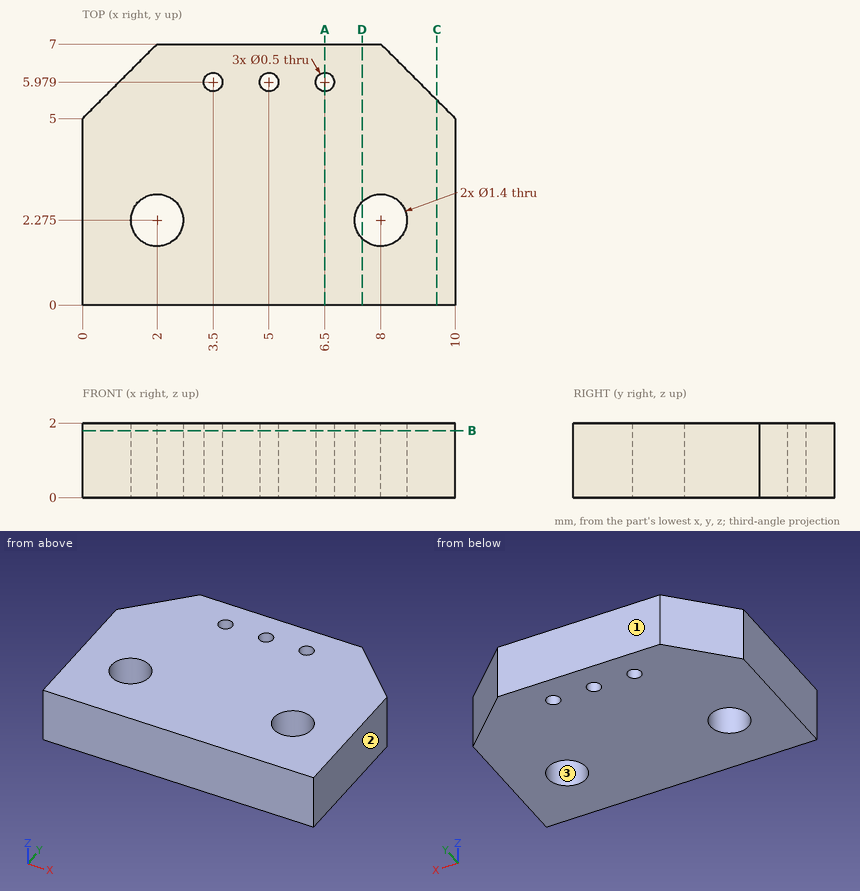
Job drawing, mm, ordinate dimensions from the low corner. One solid piece. Give positions to 0.01 mm unless a question says otherwise; leave off trailing zeros. Loops run counter-clockwise (first coordinate to the right, second up) from the corner with the lowest first, then second, coordinate; pieces in that order, holes last.
Item 1: Slice it at B-B, the plane z = 1.8. Give the number of separate pieces and of enclosed holes in the cut face.
Answers follow:
separate pieces: 1
enclosed holes: 5
Item 2: Slice it at C-C, the plane x = 9.5. List the corners of the cut face in (y, z).
Answers follow:
outline: (0, 0) - (5.5, 0) - (5.5, 2) - (0, 2) - close
Item 3: Flat gauge pin, fed straight in: pin 1 (0.8 mm diameter, centred on x = 8, y = 2.28, fed in from -Z). Where does the tip first touch, or does it go through?
Answers follow:
pin 1: passes through
Item 4: Drill centre lines: line 1 (Y direction, x = 6.5, z = 1.6); line 2 (X direction, y = 6, z = 0.6); line 3 (Y direction, x = 7.75, z = 1.25). Where is each one in solid material? Low to high.
Answers follow:
line 1: y = 0 to 5.73, 6.23 to 7
line 2: x = 1 to 3.25, 3.75 to 4.75, 5.25 to 6.25, 6.75 to 9
line 3: y = 0 to 1.62, 2.93 to 7
Item 5: Slice it at D-D, the plane x = 7.5. List the corners of the cut face in (y, z) (1 decimal).
Answers follow:
outline: (0, 0) - (1.8, 0) - (1.8, 2) - (0, 2) - close; (2.8, 0) - (7, 0) - (7, 2) - (2.8, 2) - close
Item 6: Pull direction Y, two halves, no side cores. Call the marked faces 1, 2 and 3: released by +Y, released by -Y, zero draft, split by the parting line, or undercut.
Answers follow:
face 1: released by +Y
face 2: zero draft
face 3: undercut
Item 7: Slice it at A-A, the plane x = 6.5. List the corners of the cut face in (y, z).
Answers follow:
outline: (0, 0) - (5.73, 0) - (5.73, 2) - (0, 2) - close; (6.23, 0) - (7, 0) - (7, 2) - (6.23, 2) - close
